Build history of the part. All positions in model axes, mm. A direction names the side the tool comes from. Round coordinates to 2 decimals unless told otherwise and drop trailing zeros. Loops run counter-clockwise (first coordinate to the right, second up) from the corner with the lowest first, then second, coordinate; pieces in that order, holes last. Notation, with made-up numbers: (-12, -3) - (3, -3) arc R23 cw to (3, 28) - close; hole circle Ø2 at (72, 78). An arc over 180 degrees is marked (long way). Use one line per item in the form item = value. Start each with the question number.
Q1. Pin check, flat tips, straight feed: pin 1 (3.5 mm diameter, centred on x = -5, z = -41.5, fed in from -Y); pin 2 (6 mm diameter, centred on x = -10, z = -34.5, fed in from +Y); pin 3 (2.5 mm diameter, centred on y = 51.5, z = -28, fed in from -X). Stop position of each tip, or through.
Q2. Drill centre lines: line 1 (X direction, y = 42, z = -45.25); line 2 (X direction, y = 35, z = -39.25); line 3 (Y direction, x = -5.5, z = -47.5). Where is each one in solid material? Low to high.
Q3. Saw through at B-B (y = 52.5). Give the cut face in (x, z).
Q4. Saw through at D-D (z = -45). Count the separate pieces of the cut face and the enclosed holes in it, then the cut area to 3 significant figures.
Q5. 3-axis set-ups, long thin cutter, end or side, ignore diameter. For faces 4 (the face through (-2.979, 33.637, -45.454)), 5 (the face through (-3, 32.685, -38)), 6 (the face through (-9.8, 50, -28)): which of +Z, -Z, +X, -X, +Y, -Y reach the whole face in a straight line?
Q6. Mould opens along X. For faces 1 (the face through (-8, 61, -47.7)), 2 (the face through (-1.5, 36, -42)), 3 (the face through (-7.26, 16, -45)) say: released by +X, released by -X, zero draft, split by the parting line, or undercut.
Q7. Saw through at A-A (z = -30). Give the cut face in (x, y).
Q8. Saw through at C-C (x = -1). Give the cut face in (y, z), then the cut area to 3 significant figures.
```python
from build123d import *

# Parameters (mm, degrees)
SKETCH_W        = 23
SKETCH_H        = 42
PAD_DEPTH       = 16
SKETCH001_W     = 12
SKETCH001_H     = 32
POCKET_DEPTH    = 16
SKETCH002_W     = 12
SKETCH002_H     = 4
POCKET001_DEPTH = 10
SKETCH003_W     = 6
SKETCH003_H     = 6
POCKET002_DEPTH = 11
SKETCH004_R     = 12
POCKET003_DEPTH = 1.5
SKETCH005_R     = 12
POCKET004_DEPTH = 1.5
SKETCH006_R     = 4.1
POCKET005_DEPTH = 2
SKETCH007_R     = 4.1
POCKET006_DEPTH = 2
SKETCH008_R     = 5.1
SKETCH008_R_2   = 4.1
PAD001_DEPTH    = 1
SKETCH009_R     = 5.1
SKETCH009_R_2   = 4.1
PAD002_DEPTH    = 1
SKETCH010_W     = 6
SKETCH010_H     = 8.2
POCKET007_DEPTH = 3
SKETCH011_W     = 6
SKETCH011_H     = 8.2
POCKET008_DEPTH = 3
SKETCH012_R     = 12
POCKET009_DEPTH = 6
SKETCH013_W     = 5
SKETCH013_H     = 10
POCKET010_DEPTH = 1
POCKET011_DEPTH = 16
SKETCH015_W     = 5
SKETCH015_H     = 2
POCKET012_DEPTH = 11
FILLET_R        = 3
PAD003_DEPTH    = 7
SKETCH017_W     = 0.4
SKETCH017_H     = 16
POCKET013_DEPTH = 0.4
SKETCH018_W     = 10
SKETCH018_H     = 12
PAD004_DEPTH    = 9
SKETCH019_W     = 1
SKETCH019_H     = 3
SKETCH019_W_2   = 7.000006
SKETCH019_H_2   = 7
POCKET014_DEPTH = 14.001


with BuildPart() as part:
    # Sketch → Pad (new body)
    with BuildSketch(Plane.ZY):
        with Locations((-37.200437, 34.285206)):
            Rectangle(SKETCH_W, SKETCH_H)
    extrude(amount=PAD_DEPTH)

    # Sketch001 → Pocket (cut)
    with BuildSketch(Plane.ZY.offset(16)):
        with Locations((-31.700437, 29.285206)):
            Rectangle(SKETCH001_W, SKETCH001_H)
    extrude(amount=-POCKET_DEPTH, mode=Mode.SUBTRACT)

    # Sketch002 → Pocket001 (cut)
    with BuildSketch(Plane(origin=(0, 55.285206, 0), x_dir=(0, 0, -1), z_dir=(0, 1, 0))):
        with Locations((31.700437, 2)):
            Rectangle(SKETCH002_W, SKETCH002_H)
        with Locations((31.700437, 14)):
            Rectangle(SKETCH002_W, SKETCH002_H)
        with BuildLine():
            ThreePointArc((30.700437, 6.2), (32.500437, 8), (30.700437, 9.8))
            Line((25.700437, 9.8), (30.700437, 9.8))
            Line((25.700437, 6.2), (25.700437, 9.8))
            Line((25.700437, 6.2), (30.700437, 6.2))
        make_face()
    extrude(amount=-POCKET001_DEPTH, mode=Mode.SUBTRACT)

    # Sketch003 → Pocket002 (cut)
    with BuildSketch(Plane(origin=(0, 0, -48.700437), x_dir=(0, -1, 0), z_dir=(0, 0, -1))):
        with Locations((-35.285206, 8)):
            Rectangle(SKETCH003_W, SKETCH003_H)
    extrude(amount=-POCKET002_DEPTH, mode=Mode.SUBTRACT)

    # Sketch004 → Pocket003 (cut)
    with BuildSketch(Plane.ZY.offset(5)):
        with Locations((-41.700437, 35.285206)):
            Circle(SKETCH004_R)
    extrude(amount=-POCKET003_DEPTH, mode=Mode.SUBTRACT)

    # Sketch005 → Pocket004 (cut)
    with BuildSketch(Plane(origin=(-11, 0, 0), x_dir=(0, 0, 1), z_dir=(1, 0, 0))):
        with Locations((-41.700437, -35.285206)):
            Circle(SKETCH005_R)
    extrude(amount=-POCKET004_DEPTH, mode=Mode.SUBTRACT)

    # Sketch006 → Pocket005 (cut)
    with BuildSketch(Plane.ZY.offset(3.5)):
        with Locations((-41.700437, 35.285206)):
            Circle(SKETCH006_R)
    extrude(amount=-POCKET005_DEPTH, mode=Mode.SUBTRACT)

    # Sketch007 → Pocket006 (cut)
    with BuildSketch(Plane(origin=(-12.5, 0, 0), x_dir=(0, 0, 1), z_dir=(1, 0, 0))):
        with Locations((-41.700437, -35.285206)):
            Circle(SKETCH007_R)
    extrude(amount=-POCKET006_DEPTH, mode=Mode.SUBTRACT)

    # Sketch008 → Pad001 (new body)
    with BuildSketch(Plane.ZY.offset(3.5)):
        with Locations((-41.700437, 35.285206)):
            Circle(SKETCH008_R)
        with Locations((-41.700437, 35.285206)):
            Circle(SKETCH008_R_2, mode=Mode.SUBTRACT)
    extrude(amount=PAD001_DEPTH)

    # Sketch009 → Pad002 (new body)
    with BuildSketch(Plane(origin=(-12.5, 0, 0), x_dir=(0, 0, 1), z_dir=(1, 0, 0))):
        with Locations((-41.700437, -35.285206)):
            Circle(SKETCH009_R)
        with Locations((-41.700437, -35.285206)):
            Circle(SKETCH009_R_2, mode=Mode.SUBTRACT)
    extrude(amount=PAD002_DEPTH)

    # Sketch010 → Pocket007 (cut)
    with BuildSketch(Plane.ZY.offset(4.5)):
        with Locations((-38.700437, 36.785206)):
            Rectangle(SKETCH010_W, SKETCH010_H)
    extrude(amount=-POCKET007_DEPTH, mode=Mode.SUBTRACT)

    # Sketch011 → Pocket008 (cut)
    with BuildSketch(Plane(origin=(-11.5, 0, 0), x_dir=(0, 0, 1), z_dir=(1, 0, 0))):
        with Locations((-38.700437, -36.785206)):
            Rectangle(SKETCH011_W, SKETCH011_H)
    extrude(amount=-POCKET008_DEPTH, mode=Mode.SUBTRACT)

    # Sketch012 → Pocket009 (cut)
    with BuildSketch(Plane.ZY.offset(11)):
        with Locations((-41.700437, 35.285206)):
            Circle(SKETCH012_R)
    extrude(amount=-POCKET009_DEPTH, mode=Mode.SUBTRACT)

    # Sketch013 → Pocket010 (cut)
    with BuildSketch(Plane(origin=(0, 0, -48.700437), x_dir=(0, -1, 0), z_dir=(0, 0, -1))):
        with Locations((-50.785206, 8)):
            Rectangle(SKETCH013_W, SKETCH013_H)
    extrude(amount=-POCKET010_DEPTH, mode=Mode.SUBTRACT)

    # Sketch014 → Pocket011 (cut)
    with BuildSketch(Plane.ZY.offset(16)):
        Polygon((-37.700437, 13.285206), (-48.700437, 13.285206), (-48.700437, 22.285206), (-39.700437, 22.285206), (-39.700437, 19.085206), (-41.700437, 19.085206), (-41.700437, 17.785206), (-37.700437, 17.785206), align=None)
    extrude(amount=-POCKET011_DEPTH, mode=Mode.SUBTRACT)

    # Sketch015 → Pocket012 (cut)
    with BuildSketch(Plane(origin=(0, 0, -48.700437), x_dir=(0, -1, 0), z_dir=(0, 0, -1))):
        with Locations((-52.785206, 1)):
            Rectangle(SKETCH015_W, SKETCH015_H)
        with Locations((-52.785206, 15)):
            Rectangle(SKETCH015_W, SKETCH015_H)
    extrude(amount=-POCKET012_DEPTH, mode=Mode.SUBTRACT)

    # Fillet
    fillet_edges = [part.edges().sort_by_distance(p)[0] for p in [
        (-8, 22.285206, -48.700437),
    ]]
    fillet(fillet_edges, radius=FILLET_R)

    # Sketch016 → Pad003 (new body)
    with BuildSketch(Plane(origin=(0, 0, -41.700437), x_dir=(0, -1, 0), z_dir=(0, 0, -1))):
        Polygon((-17.785206, 16), (-17.785206, 8.060191), (-14.110042, 8.060191), (-14.110042, 7.260191), (-17.785206, 7.260191), (-17.785206, 0), (-18.585206, 0), (-18.585206, 16), align=None)
    extrude(amount=PAD003_DEPTH)

    # Sketch017 → Pocket013 (cut)
    with BuildSketch(Plane(origin=(0, 18.585206, 0), x_dir=(0, 0, -1), z_dir=(0, 1, 0))):
        with Locations((41.900437, 8)):
            Rectangle(SKETCH017_W, SKETCH017_H)
    extrude(amount=-POCKET013_DEPTH, mode=Mode.SUBTRACT)

    # Sketch018 → Pad004 (new body)
    with BuildSketch(Plane(origin=(0, 55.285206, 0), x_dir=(0, 0, -1), z_dir=(0, 1, 0))):
        with Locations((43.700437, 8)):
            Rectangle(SKETCH018_W, SKETCH018_H)
    extrude(amount=PAD004_DEPTH)

    # Sketch019 → Pocket014 (cut, through all)
    with BuildSketch(Plane.ZY.offset(14)):
        with Locations((-48.200443, 60.785206)):
            Rectangle(SKETCH019_W, SKETCH019_H)
        with Locations((-42.20044, 60.785206)):
            Rectangle(SKETCH019_W_2, SKETCH019_H_2)
    extrude(amount=-POCKET014_DEPTH, mode=Mode.SUBTRACT)


solid = part.part
```
Report:
q1.pin_1 = 17.79
q1.pin_2 = 55.29
q1.pin_3 = -12
q2.line_1 = -16 to -12.5, -3.5 to 0
q2.line_2 = -16 to -14.5, -1.5 to 0
q2.line_3 = 17.79 to 18.59, 22.88 to 24.78, 45.79 to 64.29
q3.outline = (-14, -48.7) - (-13, -48.7) - (-13, -47.7) - (-3, -47.7) - (-3, -48.7) - (-2, -48.7) - (-2, -37.7) - (-4, -37.7) - (-4, -25.7) - (-6.2, -25.7) - (-6.2, -30.7) arc R1.8 cw to (-9.8, -30.7) - (-9.8, -25.7) - (-12, -25.7) - (-12, -37.7) - (-14, -37.7) - close
q4.separate_pieces = 2
q4.enclosed_holes = 1
q4.area = 326 mm²
q5.face_4 = none
q5.face_5 = +Z
q5.face_6 = +Z, +Y, -Y
q6.face_1 = zero draft
q6.face_2 = undercut
q6.face_3 = released by +X
q7.outline = (-12, 45.29) - (-9.8, 45.29) - (-9.8, 55.29) - (-12, 55.29) - close; (-6.2, 45.29) - (-4, 45.29) - (-4, 55.29) - (-6.2, 55.29) - close
q8.outline = (17.79, -48.7) - (18.59, -48.7) - (18.59, -42.1) - (18.19, -42.1) - (18.19, -41.7) - (19.09, -41.7) - (19.09, -39.7) - (22.29, -39.7) - (22.29, -45.7) arc R3 ccw to (25.29, -48.7) - (50.29, -48.7) - (50.29, -37.7) - (17.79, -37.7) - close
q8.area = 323 mm²
